```python
from build123d import *

# Parameters (mm, degrees)
SKETCH1_W           = 61
SKETCH1_H           = 100
BOSS_EXTRUDE1_DEPTH = 3
SKETCH4_W           = 61
SKETCH4_H           = 3
BOSS_EXTRUDE3_DEPTH = 10
SKETCH8_R           = 0.5
BOSS_EXTRUDE6_DEPTH = 3


with BuildPart() as part:
    # Sketch1 → Boss-Extrude1 (new body)
    with BuildSketch(Plane(origin=(0, 0, 0), x_dir=(1, 0, 0), z_dir=(0, 1, 0))):
        with Locations((30.5, 50)):
            Rectangle(SKETCH1_W, SKETCH1_H)
    extrude(amount=BOSS_EXTRUDE1_DEPTH)

    # Sketch4 → Boss-Extrude3 (add)
    with BuildSketch(Plane.XY):
        with Locations((30.5, 1.5)):
            Rectangle(SKETCH4_W, SKETCH4_H)
    extrude(amount=BOSS_EXTRUDE3_DEPTH)

    # Sketch8 → Boss-Extrude6 (add)
    with BuildSketch(Plane(origin=(61, 0, 0), x_dir=(0, 0, -1), z_dir=(1, 0, 0))):
        with BuildLine():
            Line((13.5, 3), (16.5, 3))
            Line((16.5, 3), (16.5, 5))
            ThreePointArc((16.5, 5), (15, 6.5), (13.5, 5))
            Line((13.5, 5), (13.5, 3))
        make_face()
        with Locations(Location((15, 5, 0), (0, 0, 180))):
            Circle(SKETCH8_R, mode=Mode.SUBTRACT)
    extrude(amount=-BOSS_EXTRUDE6_DEPTH)


solid = part.part
```
Check sheet for the modelled part. Datum: model origin and axes. Units: mm. A direction names the side the tool comes from. Round coordinates to 2 decimals unless told otherwise and drop trailing zeros. Order: outer loops, then holes, each group sorted by start corner. A loop starts at its lowest first (then second) coordinate and runs counter-clockwise, first axis right, second up. Notation, with made-up numbers: M -32.5,82 L -25.5,82 A27 ccw -25.5,103 Z; hole C -39.75,11 d10. An arc over 180 degrees is marked long. Answer in a Markdown table with one row per item.
(1) Section check A-A on x = 54.5. Record the boundary of the cut face in (y, z), plus the area to 3 significant figures.
Findings:
| item | result |
|---|---|
| outline | M 0,-100 L 3,-100 L 3,10 L 0,10 Z |
| area | 330 mm^2 |
(2) Set-up check for faces 1 (the flat face through (60, 4, -13.5)), 2 (the flat face through (60, 4, -16.5)), 3 (the flat face through (58, 4, -15)): record each of +Z, -Z, +X, -X, +Y, -Y from which the full face is reachable in a straight line by a thin tool's end or side.
Findings:
| item | result |
|---|---|
| face 1 | +Z, +X, -X, +Y |
| face 2 | -Z, +X, -X, +Y |
| face 3 | +Z, -Z, -X, +Y |
(3) Gauge pin test, flat ends, axial feed: pin 1 (0.6 mm diameter, centred on x = 59.5, y = 3.5, fed in from -Z); pin 2 (8 mm diameter, centred on x = 15, z = -63.5, fed in from +Y); pin 3 (3.5 mm diameter, centred on y = 5, z = -14.5, fed in from -X). Record the tip position at first contact, or that the pin passes through.
Findings:
| item | result |
|---|---|
| pin 1 | stops at z = -16.5 |
| pin 2 | stops at y = 3 |
| pin 3 | stops at x = 58 |
(4) Section check B-B on z = -74. Record the boundary of the cut face in (x, y), plus the area to 3 significant figures.
Findings:
| item | result |
|---|---|
| outline | M 0,0 L 61,0 L 61,3 L 0,3 Z |
| area | 183 mm^2 |
(5) Material ranges on line 1 along Z through (x, y) = (59.85, 5); line 2 along Y through (x, z) = (58.85, -15); line 3 along Y through (x, z) = (53, -12), recorded low to high. Write a range as from..to.
Findings:
| item | result |
|---|---|
| line 1 | z = -16.5..-15.5, -14.5..-13.5 |
| line 2 | y = 0..4.5, 5.5..6.5 |
| line 3 | y = 0..3 |
